```python
from build123d import *

# Parameters (mm, degrees)
ESQUISSE1_W                  = 69.5
ESQUISSE1_H                  = 18.6
BOSS_EXTRU_1_DEPTH           = 9.3
ENL_V_MAT_EXTRU_1_DEPTH      = 41.497067795
ENL_V_MAT_EXTRU_1_DEPTH_BACK = 41.497067795
CONG_1_R                     = 1
ESQUISSE3_R                  = 4.74
BOSS_EXTRU_2_DEPTH           = 1.45
ESQUISSE4_R                  = 4.74
BOSS_EXTRU_3_DEPTH           = 0.25
ESQUISSE5_W                  = 30
ESQUISSE5_H                  = 15
BOSS_EXTRU_4_DEPTH           = 0.1


with BuildPart() as part:
    # Esquisse1 → Boss.-Extru.1 (new body)
    with BuildSketch(Plane.XY):
        Rectangle(ESQUISSE1_W, ESQUISSE1_H)
    extrude(amount=BOSS_EXTRU_1_DEPTH)

    # Esquisse2 → Enlèv. mat.-Extru.1 (cut, two sides: drawn at the far end of the back side and taken through both)
    with BuildSketch(Plane(origin=(0, 9.3, 0), x_dir=(1, 0, 0), z_dir=(0, 1, 0)).offset(-ENL_V_MAT_EXTRU_1_DEPTH_BACK)):
        with BuildLine():
            Line((29.971199051, -6.900645436), (29.971199051, -2.399354564))
            ThreePointArc((29.971199051, -2.399354564), (31.250676471, -1.119877145), (32.53015389, -2.399354564))
            Line((32.53015389, -2.399354564), (32.53015389, -6.900645436))
            ThreePointArc((32.53015389, -6.900645436), (31.250676471, -8.180122855), (29.971199051, -6.900645436))
        make_face()
    extrude(amount=ENL_V_MAT_EXTRU_1_DEPTH + ENL_V_MAT_EXTRU_1_DEPTH_BACK, mode=Mode.SUBTRACT)

    # Congé1
    cong_1_edges = [part.edges().sort_by_distance(p)[0] for p in [
        (34.75, -9.3, 4.65),
        (-34.75, -9.3, 4.65),
        (-34.75, 9.3, 4.65),
        (34.75, 9.3, 4.65),
    ]]
    fillet(cong_1_edges, radius=CONG_1_R)

    # Esquisse3 → Boss.-Extru.2 (add)
    with BuildSketch(Plane.XY.offset(9.3)):
        with Locations(Location((25.450020764, -0.023971243, 0), (0, 0, 180))):
            Circle(ESQUISSE3_R)
    extrude(amount=BOSS_EXTRU_2_DEPTH)

    # Esquisse4 → Boss.-Extru.3 (add)
    with BuildSketch(Plane.XY.offset(9.3)):
        with Locations(Location((-25.450020764, -0.023971243, 0), (0, 0, 180))):
            Circle(ESQUISSE4_R)
    extrude(amount=BOSS_EXTRU_3_DEPTH)

    # Esquisse5 → Boss.-Extru.4 (add)
    with BuildSketch(Plane.XY.offset(9.3)):
        Rectangle(ESQUISSE5_W, ESQUISSE5_H)
    extrude(amount=BOSS_EXTRU_4_DEPTH)


solid = part.part
```
Could you check a few things on this model? Use its own coordinates, in mm. A direction names the side the tool comes from. Coordinates: 2 decimals unless noted, no trailing zeros. Write each loop counter-clockwise with the first axis right and the second up, starting at its lowest first coordinate (ties: lowest second). Pieces come first, ordered by that corner, then holes. Notation, with made-up numbers: M 38.25,72 L 49.25,72 A13 cw 49.25,93 Z; hole C 11.25,40 d2. An arc over 180 degrees is marked long. Answer as CSV lines item,"result". Start each with the question number.
1) I want a section at B-B, the plane z = 3. Please give me the cut outline in (x, y), and give its area (3 significant figures).
2) Please list where these lines run through material, in increasing order: line 1 (X direction, y = 2.25, z = 5); line 2 (Z direction, x = -12, y = 0.5); line 3 (Z direction, x = -17, y = -5.5). Write a range as from..to.
3) I want a section at D-D, the plane y = -2.75. Please give me the cut outline in (x, z).
4) We'd pull the mould along X, two halves only. Please class faces 1 (the cylindrical face through (31.28, -0.13, 8.18)), 2 (the flat face through (-34.75, 0, 5)), 3 (the flat face through (0, -9.3, 5)): +X half, -X half, draft (parallel to the pull), parting line (faces both ways), or undercut.
5) For P1, Ø5.5, axis at x = -7.5, y = -4, coming from the +Z side; P2, Ø4.5, axis at x = -24.5, y = -1.5, coming from the +Z side, each with a flat end and sliding along its axis, tell me the tip position at first contact or that it passes through.
6) I want a section at C-C, the plane x = -9. Please give me the cut outline in (y, z), and give its area (3 significant figures).
7) I want a section at A-A, the plane y = 6.25. Please give me the cut outline in (x, z).
8) For faces 4 (the cylindrical face through (20.93, -1.45, 10.01)), 5 (the cylindrical face through (31.22, -0.13, 1.12)), 6 (the flat face through (0, 0, 9.4)), 7 (the flat face through (-25, 0, 9.55)), which set-ups out of +Z, -Z, +X, -X, +Y, -Y let a thin tool reach every point of the face, with its end or its side?
Data:
1,outline,"M -34.75,-8.3 A1 ccw -33.75,-9.3 L 29.97,-9.3 L 29.97,9.3 L -33.75,9.3 A1 ccw -34.75,8.3 Z; M 32.53,-9.3 L 33.75,-9.3 A1 ccw 34.75,-8.3 L 34.75,8.3 A1 ccw 33.75,9.3 L 32.53,9.3 Z"
1,area,"1,240 mm^2"
2,line 1,"x = -34.75..29.97, 32.53..34.75"
2,line 2,"z = 0..9.4"
2,line 3,"z = 0..9.3"
3,outline,"M -34.75,0 L 34.75,0 L 34.75,9.3 L 29.33,9.3 L 29.33,10.75 L 21.57,10.75 L 21.57,9.3 L 15,9.3 L 15,9.4 L -15,9.4 L -15,9.3 L -21.57,9.3 L -21.57,9.55 L -29.33,9.55 L -29.33,9.3 L -34.75,9.3 Z; hole M 29.97,2.4 A1.28 ccw 32.53,2.4 L 32.53,6.9 A1.28 ccw 29.97,6.9 Z"
4,face 1,"undercut"
4,face 2,"-X half"
4,face 3,"draft"
5,P1,"stops at z = 9.4"
5,P2,"stops at z = 9.55"
6,outline,"M -9.3,0 L 9.3,0 L 9.3,9.3 L 7.5,9.3 L 7.5,9.4 L -7.5,9.4 L -7.5,9.3 L -9.3,9.3 Z"
6,area,"174 mm^2"
7,outline,"M -34.75,0 L 34.75,0 L 34.75,9.3 L 15,9.3 L 15,9.4 L -15,9.4 L -15,9.3 L -34.75,9.3 Z; hole M 29.97,2.4 A1.28 ccw 32.53,2.4 L 32.53,6.9 A1.28 ccw 29.97,6.9 Z"
8,face 4,"+Z"
8,face 5,"+Y, -Y"
8,face 6,"+Z, +Y, -Y"
8,face 7,"+Z, -X, +Y, -Y"
